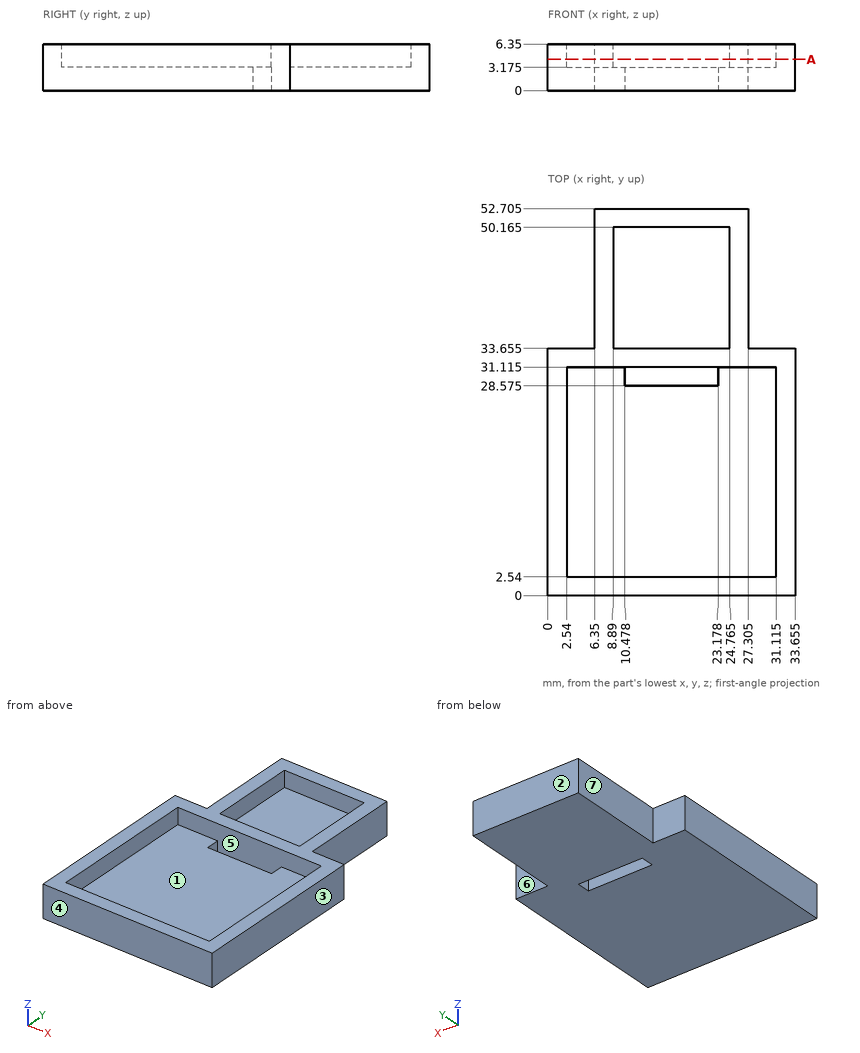
Check sheet for the drawn part. Datum: minimum x, y, z corner. Units: mm. A direction names the side the tool comes from. Round coordinates to 2 decimals unless told otherwise and drop trailing zeros.
Item 1: Thickness scan on line 1 (Y direction, x = 18.5, z = 5) (1 decimal); line 2 (Y direction, x = 13, z = 0.5) (1 decimal); line 3 (Y direction, x = 7, z = 4.75) (1 decimal). Record the ranges inside material, lowest first.
Item 2: Mould release check, pull along Y, two halves, no side actions. Record for the marked faces 1, 2, 3 and 4: pulls with the +Y half, pulls with the -Y half, needs draft (parallel to the pull), parting line crosses it, or undercut.
Item 3: Gauge pin test, flat ends, axial feed: pin 1 (1 mm diameter, centred on x = 23, y = 15, fed in from +Z) (1 decimal); pin 2 (1.9 mm diameter, centred on y = 41.5, z = 3, fed in from +X) (1 decimal); pin 3 (1 mm diameter, centred on y = 42, z = 4.5, fed in from -X). Record the tip position at first contact, or that the pin passes through.
Item 4: Access from +Z, -Z, +X, -X, +Y, -Y to the whole of each face (thin tool, end or side, straight path). Record for the marked faces 5, 6 and 7.
Item 5: Cross-section at A-A on z = 4.25. Count the separate pieces of the cut face and the enclosed holes in it.
Answer sheet:
1. line 1: y = 0 to 2.5, 31.1 to 33.7, 50.2 to 52.7
1. line 2: y = 0 to 28.6, 31.1 to 52.7
1. line 3: y = 0 to 2.5, 31.1 to 52.7
2. face 1: undercut
2. face 2: pulls with the +Y half
2. face 3: needs draft
2. face 4: pulls with the -Y half
3. pin 1: stops at z = 3.2
3. pin 2: stops at x = 27.3
3. pin 3: stops at x = 6.35
4. face 5: +Z
4. face 6: +Z, -Z, +X, +Y
4. face 7: +Z, -Z, -X, +Y
5. separate pieces: 1
5. enclosed holes: 2
